Build history of the part. All positions in model axes, mm. A direction names the side the tool comes from. Round coordinates to 2 decimals unless told otherwise and drop trailing zeros. Loops run counter-clockwise (first coordinate to the right, second up) from the corner with the lowest first, then second, coordinate; pieces in that order, holes last. Notation, with made-up numbers: (34, 68) - (82, 68) arc R18 ccw to (82, 93) - close; hole circle Ø5 at (80.5, -9). An arc over 180 degrees is marked (long way). Use a Markdown table: item, result.
from build123d import *

# Parameters (mm, degrees)
F0_R     = 9
F1_DEPTH = 100
F2_R     = 9
F2_R_2   = 8
F3_DEPTH = 42
F4_R     = 8.975
F5_DEPTH = 10
F7_D     = 16


# Not quite as in the source:
# - a fillet or chamfer that OpenCascade refuses, or shapes differently, is made with other operations: its cross-section is extruded or revolved along the edge and cut away or added


with BuildPart() as f1:
    # F0 (on Top) → F1 (new body)
    with BuildSketch(Plane.XY):
        with BuildLine():
            Line((11.6741448398, 1.375), (12.4241448398, 1.375))
            ThreePointArc((12.4241448398, 1.375), (8.8388347648, 8.8388347648), (1.375, 12.4241448398))
            Line((1.375, 12.4241448398), (1.375, 11.6741448398))
            Line((1.375, 11.6741448398), (-1.375, 11.6741448398))
            Line((-1.375, 11.6741448398), (-1.375, 12.4241448398))
            ThreePointArc((-1.375, 12.4241448398), (-8.8388347648, 8.8388347648), (-12.4241448398, 1.375))
            Line((-12.4241448398, 1.375), (-11.6741448398, 1.375))
            Line((-11.6741448398, 1.375), (-11.6741448398, -1.375))
            Line((-11.6741448398, -1.375), (-12.4241448398, -1.375))
            ThreePointArc((-12.4241448398, -1.375), (-8.8388347648, -8.8388347648), (-1.375, -12.4241448398))
            Line((-1.375, -12.4241448398), (-1.375, -11.6741448398))
            Line((-1.375, -11.6741448398), (1.375, -11.6741448398))
            Line((1.375, -11.6741448398), (1.375, -12.4241448398))
            ThreePointArc((1.375, -12.4241448398), (8.8388347648, -8.8388347648), (12.4241448398, -1.375))
            Line((12.4241448398, -1.375), (11.6741448398, -1.375))
            Line((11.6741448398, -1.375), (11.6741448398, 1.375))
        make_face()
        Circle(F0_R, mode=Mode.SUBTRACT)
    extrude(amount=F1_DEPTH)

    # F2 (on Top) → F3 (join)
    with BuildSketch(Plane.XY):
        Circle(F2_R)
        Circle(F2_R_2, mode=Mode.SUBTRACT)
    extrude(amount=F3_DEPTH)

    # F4 (on Top) → F5 (join)
    with BuildSketch(Plane.XY):
        Circle(F4_R)
    extrude(amount=-F5_DEPTH)

    # F7 (through all)
    with Locations(Plane(origin=(0, 0, -10), x_dir=(1, 0, 0), z_dir=(0, 0, -1))):
        with Locations((0, 0)):
            Hole(F7_D / 2)

    # F8: chamfer of 1 on 1 edges, made by hand

    # F8_s1 → F8_t2 (revolve, cut)
    with BuildSketch(Plane.XZ):
        Polygon((8.975, -9), (7.975, -10), (8.975, -10), align=None)
    revolve(axis=Axis((0, 0, -10), (0, 0, 1)), mode=Mode.SUBTRACT)


solid = f1.part
Q1. Cut at A-A, the plane z = 58.5. List the corners of the cut face in (x, y) (3 decimals), plus the area to 3 significant figures.
Results found:
| item | result |
|---|---|
| outline | (-12.424, -1.375) arc R12.5 ccw to (-1.375, -12.424) - (-1.375, -11.674) - (1.375, -11.674) - (1.375, -12.424) arc R12.5 ccw to (12.424, -1.375) - (11.674, -1.375) - (11.674, 1.375) - (12.424, 1.375) arc R12.5 ccw to (1.375, 12.424) - (1.375, 11.674) - (-1.375, 11.674) - (-1.375, 12.424) arc R12.5 ccw to (-12.424, 1.375) - (-11.674, 1.375) - (-11.674, -1.375) - close; hole circle Ø18 at (0, 0) |
| area | 228 mm2 |
Q2. Pull direction X, two halves, no side cores. Call faces 5 (the face through (-8.922, -8.755, 49.3)), 6 (the face through (-1.172, 8.923, 70.594)), 7 (the face through (8.755, -8.922, 49.3)): pulls with the +X half, pulls with the -X half, needs draft (parallel to the pull), parting line crosses it, or undercut.
Results found:
| item | result |
|---|---|
| face 5 | pulls with the -X half |
| face 6 | undercut |
| face 7 | pulls with the +X half |
Q3. Cut at D-D, the plane z = -1. List the corners of the cut face in (x, y) (3 decimals), plus the area to 3 significant figures.
Results found:
| item | result |
|---|---|
| outline | circle Ø17.95 at (0, 0); hole circle Ø16 at (0, 0) |
| area | 52.0 mm2 |
Q4. Which spindle directions (+Z, -Z, +X, -X, +Y, -Y) get a long thin tool onto all of the face, cutting with end or side? Do faces 1 (the face through (0, 11.674, 49)), 2 (the face through (8, -5, 0)), 3 (the face through (11.674, 0, 49)), 4 (the face through (0, -11.674, 49)). Say none if no direction does.
Results found:
| item | result |
|---|---|
| face 1 | +Z, -Z, +Y |
| face 2 | -Z |
| face 3 | +Z, -Z, +X |
| face 4 | +Z, -Z, -Y |
Q5. Probe line 1 (Y direction, x = 0, z = -7.5) (3 decimals); line 2 (Y direction, x = 0, z = 65); line 3 (Z direction, x = -1, y = 11.25). List the from-to ranges inside material, lowest first.
Results found:
| item | result |
|---|---|
| line 1 | y = -8.975 to -8, 8 to 8.975 |
| line 2 | y = -11.67 to -9, 9 to 11.67 |
| line 3 | z = 0 to 100 |
Q6. Cut at B-B, the plane x = 0. List the corners of the cut face in (y, z) (3 decimals).
Results found:
| item | result |
|---|---|
| outline | (-11.674, 0) - (-8.975, 0) - (-8.975, -9) - (-8, -9.975) - (-8, 42) - (-9, 42) - (-9, 100) - (-11.674, 100) - close; (8, -9.975) - (8.975, -9) - (8.975, 0) - (11.674, 0) - (11.674, 100) - (9, 100) - (9, 42) - (8, 42) - close |
Q7. Drop flat-ended pins along their axis: pin 1 (0.8 mm diameter, centred on x = -0.5, z = 43.5, fed in from +Y); pin 2 (0.8 mm diameter, centred on y = -12, z = 36.5, fed in from -X); pin 3 (2 mm diameter, centred on x = 0, z = 41.5, fed in from -Y); pin 4 (14.5 mm diameter, centred on x = 0, y = 0, fed in from +Z). Give the stop position or say it passes through.
Results found:
| item | result |
|---|---|
| pin 1 | stops at y = 11.67 |
| pin 2 | stops at x = -4.66 |
| pin 3 | stops at y = -11.67 |
| pin 4 | passes through |
Q8. Cut at C-C, the plane y = 10. List the corners of the cut face in (x, z), plus the area to 3 significant figures.
Results found:
| item | result |
|---|---|
| outline | (-7.5, 0) - (7.5, 0) - (7.5, 100) - (-7.5, 100) - close |
| area | 1,500 mm2 |
